Could you check a few things on this drawing? It's one solid part, dimensions in mm from its lowest x, y, z. Give positions to 0.01 mm unless a question says otherwise; leave off trailing zeros. Order: outer loops, then holes, each group sorted by start corner. A loop starts at its lowest first (then second) coordinate and runs counter-clockwise, first axis right, second up. Notation, with made-up numbers: M 7,89 L 30,89 A23 cw 30,114 Z; hole C 89.5,89.5 d2. An arc over 180 degrees is marked long. Use one line per item in the form item = value.
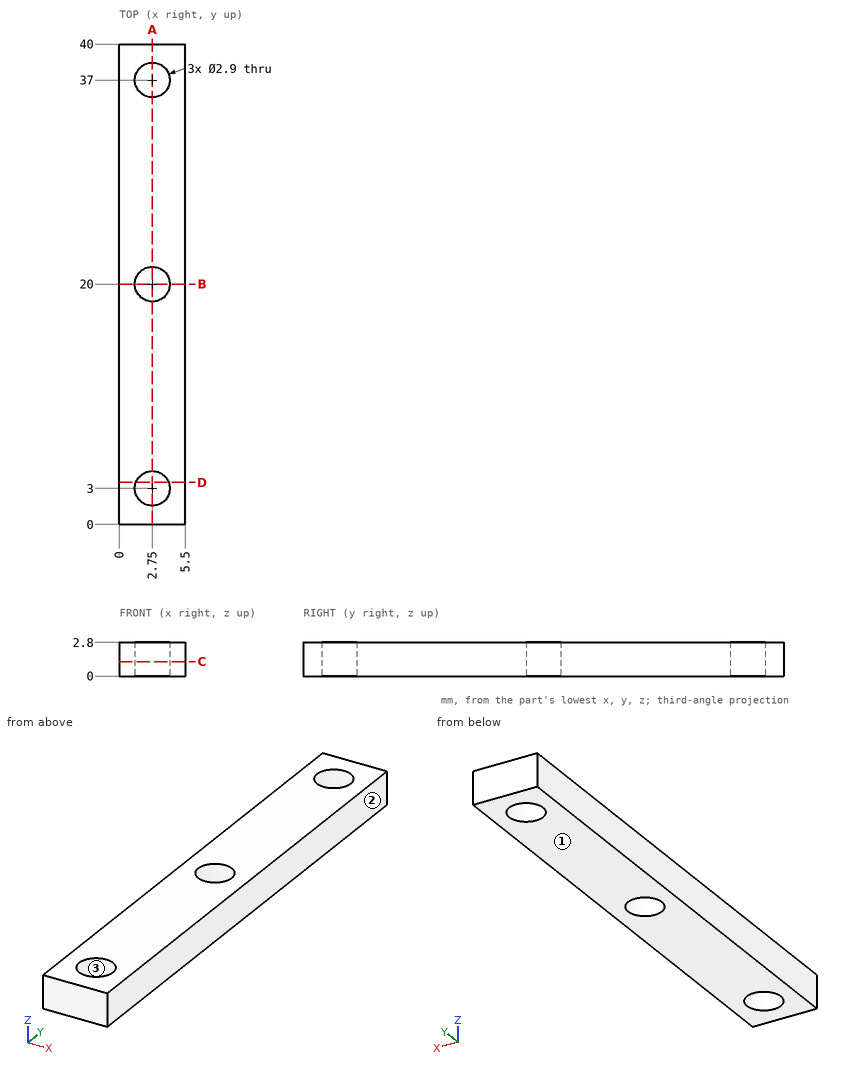
Q1. I want a section at B-B on y = 20. Write out the boundary of the cut face in (x, z).
Found:
outline = M 0,0 L 1.3,0 L 1.3,2.8 L 0,2.8 Z; M 4.2,0 L 5.5,0 L 5.5,2.8 L 4.2,2.8 Z
Q2. Thinking about a two-plate mould opening in X: for the marked faces 1, 2 and 3, which applies, +X half, -X half, draft (parallel to the pull), parting line (faces both ways), or undercut?
Found:
face_1 = draft
face_2 = +X half
face_3 = undercut
Q3. I want a section at A-A on x = 2.75. Write out the boundary of the cut face in (y, z).
Found:
outline = M 0,0 L 1.55,0 L 1.55,2.8 L 0,2.8 Z; M 4.45,0 L 18.55,0 L 18.55,2.8 L 4.45,2.8 Z; M 21.45,0 L 35.55,0 L 35.55,2.8 L 21.45,2.8 Z; M 38.45,0 L 40,0 L 40,2.8 L 38.45,2.8 Z
Q4. I need wall thicknesses on L1, parallel to Y at x = 2.75, z = 0.7; L2, parallel to X at y = 21, z = 0.1. Which ranges of each line are inside material? Lowest first, please.
Found:
L1 = 0 to 1.55, 4.45 to 18.55, 21.45 to 35.55, 38.45 to 40
L2 = 0 to 1.7, 3.8 to 5.5
Q5. I want a section at C-C on z = 1.2. Write out the boundary of the cut face in (x, y), then the cut area to 3 significant figures.
Found:
outline = M 0,0 L 5.5,0 L 5.5,40 L 0,40 Z; hole C 2.75,3 d2.9; hole C 2.75,20 d2.9; hole C 2.75,37 d2.9
area = 200 mm²
Q6. I want a section at D-D on y = 3.5. Write out the boundary of the cut face in (x, z).
Found:
outline = M 0,0 L 1.39,0 L 1.39,2.8 L 0,2.8 Z; M 4.11,0 L 5.5,0 L 5.5,2.8 L 4.11,2.8 Z
